```python
from build123d import *

# Parameters (mm, degrees)
F0_R     = 13.5
F0_R_2   = 10
F1_DEPTH = 15
F2_R     = 12.75
F3_DEPTH = 13.5
F4_SIZE  = 0.75


with BuildPart() as f1:
    # F0 (on Top) → F1 (new body)
    with BuildSketch(Plane.XY):
        Circle(F0_R)
        Circle(F0_R_2, mode=Mode.SUBTRACT)
    extrude(amount=F1_DEPTH)

    # F2 (on face) → F3 (cut)
    with BuildSketch(Plane.XY.offset(15)):
        Circle(F2_R)
    extrude(amount=-F3_DEPTH, mode=Mode.SUBTRACT)

    # F4
    f4_edges = [f1.edges().sort_by_distance(p)[0] for p in [
        (-13.5, 0, 0),
        (-10, 0, 0),
    ]]
    chamfer(f4_edges, length=F4_SIZE)


solid = f1.part
```
Read the model definition and answer for the solid it produces. Units are mm, in the model's axes. A direction names the side the tool comes from. Give positions to 0.01 mm unless a question says otherwise; leave off trailing zeros. Write each loop counter-clockwise with the first axis right and the second up, starting at its lowest first coordinate (ties: lowest second). Pieces come first, ordered by that corner, then holes. Notation, with made-up numbers: (43, 37) - (48, 37) arc R24 cw to (48, 58) - close; hole circle Ø1 at (44, 1). An arc over 180 degrees is marked (long way). Write item = value, one per line. Start each with the question number.
Item 1: Find section C-C (z = 13). Give the vertices of the cut face in (x, y), then the cut area to 4 significant figures.
Item 2: The mould has two halves that part along Y. Classify faces 1 (the flat face through (-5.7, -9.4, 0)), 2 (the cylindrical face through (-2.764, -12.447, 8.344)), 3 (the cylindrical face through (-2.93, -13.18, 7.78)): +Y half, -Y half, draft (parallel to the pull), parting line (faces both ways), or undercut.
Item 3: Each of these flat-tipped pins is pushed along its axis until it touches: P1, Ø2, axis at x = -8.5, z = 8.5, coming from the +Y side (3 decimals); P2, Ø6, axis at x = -4.5, y = -5.5, coming from the +Z side. Where does it stop, or does it pass through?
Item 4: Find the intervals of material crossed by probe 1 along Y at (x, z) = (0, 7); probe 2 along Y at (x, z) = (0, 1); probe 3 along Z at (x, y) = (-3, -11.75), in increasing order. Write a range as [from, to].
Item 5: Find section A-A (x = 0). Give the vertices of the cut face in (y, z), then the cut area to 3 significant figures.
Item 6: A tool of negligible diameter and unlimited length cuts with its end or side. For faces 4 (the flat face through (-8, -7, 1.5)), 5 (the cylindrical face through (-2.17, -9.76, 1.12)), from which of +Z, -Z, +X, -X, +Y, -Y can it reach the whole face along a straight path? Write none if from no direction.
Response:
q1.outline = circle Ø27 at (0, 0); hole circle Ø25.5 at (0, 0)
q1.area = 61.85 mm²
q2.face_1 = draft
q2.face_2 = undercut
q2.face_3 = parting line
q3.P1 = 11.225
q3.P2 = 1.5
q4.probe_1 = [-13.5, -12.75], [12.75, 13.5]
q4.probe_2 = [-13.5, -10], [10, 13.5]
q4.probe_3 = [0, 1.5]
q5.outline = (-13.5, 0.75) - (-12.75, 0) - (-10.75, 0) - (-10, 0.75) - (-10, 1.5) - (-12.75, 1.5) - (-12.75, 15) - (-13.5, 15) - close; (10, 0.75) - (10.75, 0) - (12.75, 0) - (13.5, 0.75) - (13.5, 15) - (12.75, 15) - (12.75, 1.5) - (10, 1.5) - close
q5.area = 29.6 mm²
q6.face_4 = +Z
q6.face_5 = +Z, -Z
